```python
from build123d import *

# Parameters (mm, degrees)
CROQUIS1_R              = 2.5
SALIENTE_EXTRUIR1_DEPTH = 3


with BuildPart() as part:
    # Croquis1 → Saliente-Extruir1 (new body)
    with BuildSketch(Plane.XY):
        Polygon((-45, 0), (45, 0), (37.720595315, 20), (-37.720595315, 20), align=None)
        with Locations((-30, 10)):
            Circle(CROQUIS1_R, mode=Mode.SUBTRACT)
        with Locations((30, 10)):
            Circle(CROQUIS1_R, mode=Mode.SUBTRACT)
    extrude(amount=SALIENTE_EXTRUIR1_DEPTH)


solid = part.part
```
Check sheet for the modelled part. Datum: model origin and axes. Units: mm. Coordinates: 2 decimals unless noted, no trailing zeros. Order: outer loops, then holes, each group sorted by start corner. A loop starts at its lowest first (then second) coordinate and runs counter-clockwise, first axis right, second up. Notation, with made-up numbers: (-19.75, -22) -> (8.25, -22) arc R11 ccw to (8.25, -7) -> close; hole circle Ø4 at (76, 71). An arc over 180 degrees is marked (long way). Write item = value, one per line. Start each with the question number.
1) Mould release check, pull along Y, two halves, no side actions. Record for faces 1 (the cylindrical face through (29.46, 7.56, 1.48)), 2 (the flat face through (-1, 10, 0)), 3 (the flat face through (41.41, 9.86, 1.48)): +Y half, -Y half, draft (parallel to the pull), parting line (faces both ways), or undercut.
2) Cross-section at C-C (y = 10). Enter the section's corners in (x, z), then the cut area to 3 significant figures.
3) Cross-section at A-A (x = -31.5). Enter the section's corners in (y, z).
4) Cross-section at B-B (z = 1.5). Enter the section's corners in (x, y).
5) Cross-section at D-D (x = 30). Enter the section's corners in (y, z).
6) Go/stop test with a flat-tipped pin: P1, Ø6.5, axis at x = 30, y = 10, coming from the +Z side. Record where the tip stops, or that it passes through.
7) Material ranges on L1, parallel to X at y = 10.25, z = 1.2; L2, parallel to Y at x = 30, z = 1; L3, parallel to Y at x = -29, z = 2.75, recorded low to high.
Ans:
q1.face_1 = undercut
q1.face_2 = draft
q1.face_3 = +Y half
q2.outline = (-41.36, 0) -> (-32.5, 0) -> (-32.5, 3) -> (-41.36, 3) -> close; (-27.5, 0) -> (27.5, 0) -> (27.5, 3) -> (-27.5, 3) -> close; (32.5, 0) -> (41.36, 0) -> (41.36, 3) -> (32.5, 3) -> close
q2.area = 218 mm²
q3.outline = (0, 0) -> (8, 0) -> (8, 3) -> (0, 3) -> close; (12, 0) -> (20, 0) -> (20, 3) -> (12, 3) -> close
q4.outline = (-45, 0) -> (45, 0) -> (37.72, 20) -> (-37.72, 20) -> close; hole circle Ø5 at (-30, 10); hole circle Ø5 at (30, 10)
q5.outline = (0, 0) -> (7.5, 0) -> (7.5, 3) -> (0, 3) -> close; (12.5, 0) -> (20, 0) -> (20, 3) -> (12.5, 3) -> close
q6.P1 = 3
q7.L1 = -41.27 to -32.49, -27.51 to 27.51, 32.49 to 41.27
q7.L2 = 0 to 7.5, 12.5 to 20
q7.L3 = 0 to 7.71, 12.29 to 20
